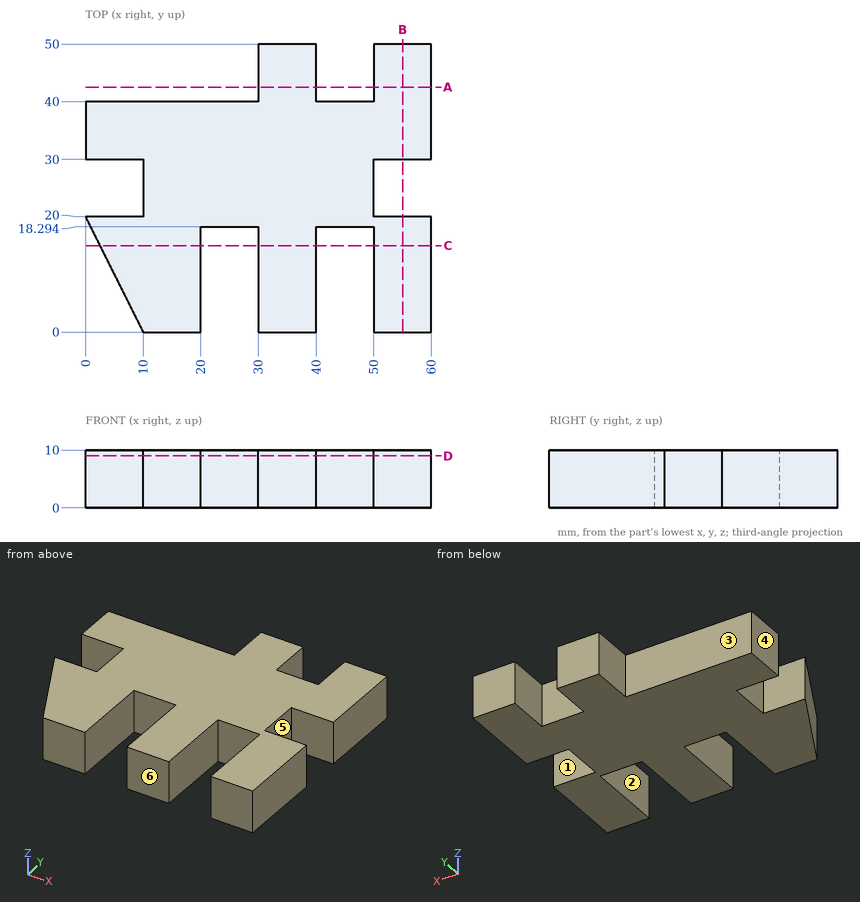
Could you check a few things on this drawing? It's one solid part, dimensions in mm from its lowest x, y, z. A direction names the side the tool comes from. Coordinates: 2 decimals unless noted, no trailing zeros. Order: outer loops, then holes, each group sorted by start corner. A loop starts at its lowest first (then second) coordinate and runs counter-clockwise, first axis right, second up.
1. Thinking about a two-plate mould opening in Y: for the marked faces 4, 5 and 6, which applies, +Y half, -Y half, draft (parallel to the pull), parting line (faces both ways), or undercut?
2. If we section it at A-A (y = 42.5): Please give me the cut outline in (x, z).
3. I'm going to push flat-ended pins straight in: pin 1 (1.5 mm diameter, centred on x = 29, y = 8.5, fed in from +Z); pin 2 (5 mm diameter, centred on y = 5, z = 5.5, fed in from -X); pin 3 (5 mm diameter, centred on x = 7, z = 2, fed in from -Y); pin 4 (1.5 mm diameter, centred on x = 14, z = 2, fed in from +Y). Where does each tip first touch, or does it pass through?
4. If we section it at D-D (z = 9): Please give me the cut outline in (x, y).
5. For the marked faces 1, 2 and 3, which set-ups out of +Z, -Z, +X, -X, +Y, -Y let a thin tool reach every point of the face, with its end or its side?
6. If we section it at C-C (y = 15): Please give me the cut outline in (x, z).
7. If we section it at B-B (x = 55): Please give me the cut outline in (y, z), then the cut area to 3 significant figures.
8. I need wall thicknesses on line 1 (Y direction, x = 55, z = 5); line 2 (X direction, y = 3, z = 7.5); line 3 (X direction, y = 8, z = 5). Which ranges of each line are inside material? Lowest first, please.
Entries:
1. face 4: draft
1. face 5: undercut
1. face 6: -Y half
2. outline: (30, 0) - (40, 0) - (40, 10) - (30, 10) - close; (50, 0) - (60, 0) - (60, 10) - (50, 10) - close
3. pin 1: passes through
3. pin 2: stops at x = 6.25
3. pin 3: stops at y = 1
3. pin 4: stops at y = 40
4. outline: (0, 20) - (10, 0) - (20, 0) - (20, 18.29) - (30, 18.29) - (30, 0) - (40, 0) - (40, 18.29) - (50, 18.29) - (50, 0) - (60, 0) - (60, 20) - (50, 20) - (50, 30) - (60, 30) - (60, 50) - (50, 50) - (50, 40) - (40, 40) - (40, 50) - (30, 50) - (30, 40) - (0, 40) - (0, 30) - (10, 30) - (10, 20) - close
5. face 1: +Z, -Z, +X
5. face 2: +Z, -Z, -Y
5. face 3: +Z, -Z, -X, +Y
6. outline: (2.5, 0) - (20, 0) - (20, 10) - (2.5, 10) - close; (30, 0) - (40, 0) - (40, 10) - (30, 10) - close; (50, 0) - (60, 0) - (60, 10) - (50, 10) - close
7. outline: (0, 0) - (20, 0) - (20, 10) - (0, 10) - close; (30, 0) - (50, 0) - (50, 10) - (30, 10) - close
7. area: 400 mm2
8. line 1: y = 0 to 20, 30 to 50
8. line 2: x = 8.5 to 20, 30 to 40, 50 to 60
8. line 3: x = 6 to 20, 30 to 40, 50 to 60
